Design review of the part built by this model. Coordinates are the model's own, in mm. A direction names the side the tool comes from. Round coordinates to 2 decimals unless told otherwise and drop trailing zeros. Order: outer loops, then holes, each group sorted by start corner. A loop starts at its lowest first (then second) coordinate and runs counter-clockwise, first axis right, second up.
from build123d import *

# Parameters (mm, degrees)
SKETCH2_R           = 4
SKETCH2_R_2         = 2.5
BOSS_EXTRUDE1_DEPTH = 4
SKETCH3_W           = 24
SKETCH3_H           = 48
BOSS_EXTRUDE2_DEPTH = 15
SKETCH4_W           = 20
SKETCH4_H           = 40
CUT_EXTRUDE1_DEPTH  = 15
FILLET1_R           = 3


with BuildPart() as part:
    # Sketch2 → Boss-Extrude1 (new body)
    # profile 1 of 2: a face of its own
    with BuildSketch(Plane(origin=(0, 0, 0), x_dir=(0, 0, -1), z_dir=(1, 0, 0))):
        with Locations((0, 1)):
            Circle(SKETCH2_R)
        with Locations((0, 1)):
            Circle(SKETCH2_R_2, mode=Mode.SUBTRACT)
    # profile 2 of 2: a face of its own
    with BuildSketch(Plane(origin=(0, 0, 0), x_dir=(0, 0, -1), z_dir=(1, 0, 0))):
        with BuildLine():
            Line((-4, 1), (-4, -5))
            Line((-4, -5), (4, -5))
            Line((4, -5), (4, 1))
            ThreePointArc((4, 1), (0, -3), (-4, 1))
        make_face()
    extrude(amount=BOSS_EXTRUDE1_DEPTH)

    # Sketch3 → Boss-Extrude2 (add)
    with BuildSketch(Plane(origin=(4, 0, 0), x_dir=(0, 0, -1), z_dir=(1, 0, 0))):
        with Locations((8, -29)):
            Rectangle(SKETCH3_W, SKETCH3_H)
    extrude(amount=-BOSS_EXTRUDE2_DEPTH)

    # Sketch4 → Cut-Extrude1 (cut)
    with BuildSketch(Plane.ZY.offset(11)):
        with Locations((-10, -29)):
            Rectangle(SKETCH4_W, SKETCH4_H)
    extrude(amount=-CUT_EXTRUDE1_DEPTH, mode=Mode.SUBTRACT)

    # Fillet1
    fillet1_edges = [part.edges().sort_by_distance(p)[0] for p in [
        (-3.5, -9, -20),
        (-3.5, -49, -20),
    ]]
    fillet(fillet1_edges, radius=FILLET1_R)


solid = part.part
1) To check wall thickness, follow line 1 along Y through (x, z) = (-6, -14.5); line 2 along Z through (x, y) = (3.25, -17.5). State the ranges of each line that lie inside material, in increasing order.
Results:
line 1: y = -53 to -49, -9 to -5
line 2: z = 0 to 4
2) Clearance check with flat-ended pins moving along their axes: P1, Ø6, axis at y = 1, z = 0, coming from the -X side; P2, Ø1.2, axis at x = 3, y = -2, coming from the -Z side; P3, Ø2.5, axis at y = 1, z = -1, coming from the -X side; P4, Ø2, axis at x = -4.5, z = -1.5, coming from the +Y side. State where each tip first meets the part, or that it passes through.
Results:
P1: stops at x = 0
P2: stops at z = -4
P3: passes through
P4: stops at y = -5
3) For faces 1 (the face through (2, -2, -4)), 2 (the face through (-3.39, -49.9, -19.14)), 3 (the face through (-3.4, -52.5, -20)), 4 (the face through (0, -2, 0)), list the 3-axis set-ups (+Z, -Z, +X, -X, +Y, -Y) from which the entire face can be reached by the end or side of a thin tool; tool diameter is ignored.
Results:
face 1: -Z, +X, -X, +Y
face 2: -Z, +X, -X
face 3: -Z, +X, -X, +Y, -Y
face 4: +Z, -Z, -X, +Y
4) Take a section at A-A on z = -6.25. Give the boundary of the cut face in (x, y), plus the area to 3 significant figures.
Results:
outline: (-11, -53) - (4, -53) - (4, -49) - (-11, -49) - close; (-11, -9) - (4, -9) - (4, -5) - (-11, -5) - close
area: 120 mm2
5) The part is to be moulded in two halves that separate along Y. For faces 5 (the face through (1.97, 3.48, 0.33)), 6 (the face through (2, 5, 0)), 7 (the face through (-3, -26, 4)), say which applies: released by +Y, released by -Y, zero draft, split by the parting line, or undercut.
Results:
face 5: undercut
face 6: released by +Y
face 7: zero draft
6) Take a section at B-B on x = -8. Give the boundary of the cut face in (y, z).
Results:
outline: (-53, -20) - (-52, -20) arc R3 ccw to (-49, -17) - (-49, 0) - (-9, 0) - (-9, -17) arc R3 ccw to (-6, -20) - (-5, -20) - (-5, 4) - (-53, 4) - close
7) Take a section at C-C on y = -47.5. Give the boundary of the cut face in (x, z).
Results:
outline: (-11, 0) - (4, 0) - (4, 4) - (-11, 4) - close
